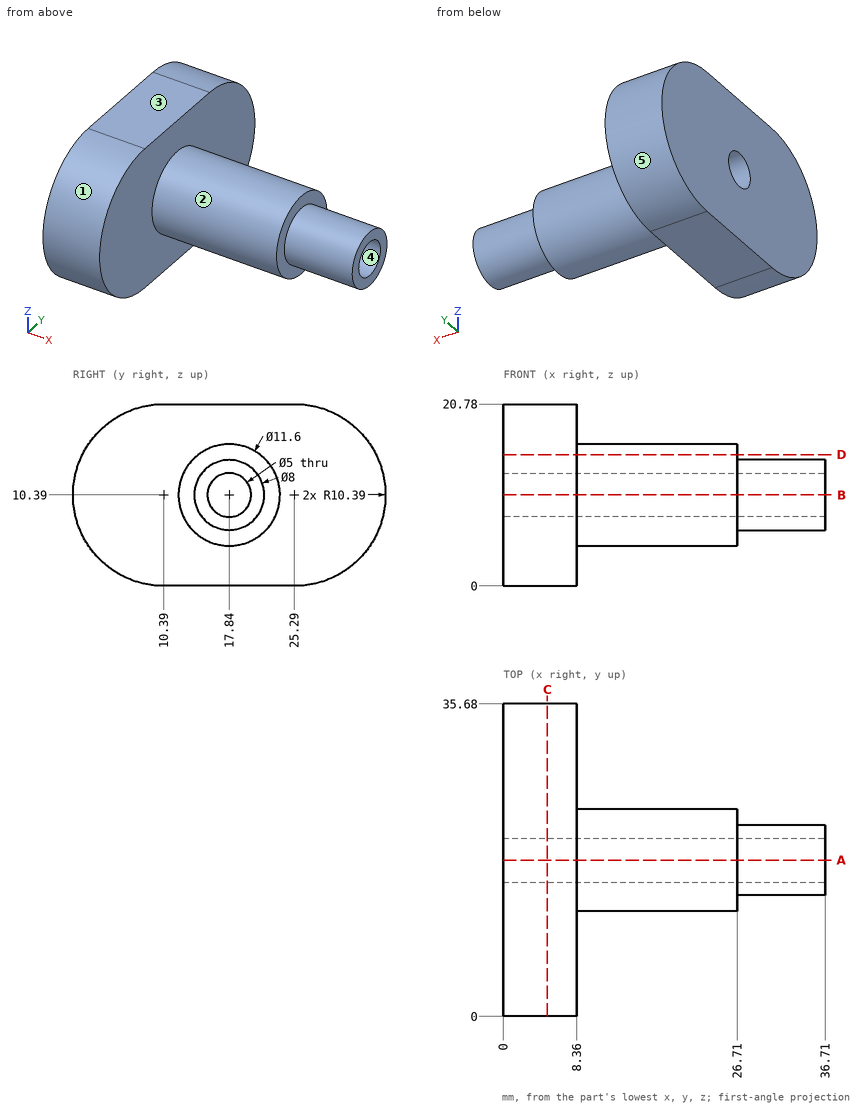
Check sheet for the drawn part. Datum: minimum x, y, z corner. Units: mm. A direction names the side the tool comes from. Coordinates: 2 decimals unless noted, no trailing zeros. Order: outer loops, then holes, each group sorted by start corner. A loop starts at its lowest first (then second) coordinate and runs counter-clockwise, first axis right, second up. Notation, with made-up numbers: (-11.5, 71) -> (39.5, 71) arc R30 cw to (39.5, 98) -> close; hole circle Ø2 at (82.5, 3). An arc over 180 degrees is marked (long way). Use a Markdown table: item, result. Add a question column.
1. Cross-section at C-C (x = 5). Enter the section's corners in (y, z).
2. Set-up check for the marked faces 1 and 2: record each of +Z, -Z, +X, -X, +Y, -Y from which the full face is reachable in a straight line by a thin tool's end or side.
3. Cross-section at A-A (y = 17.84). Enter the section's corners in (x, z).
4. Cross-section at D-D (z = 15). Enter the section's corners in (x, y).
5. Cross-section at B-B (z = 10.39). Enter the section's corners in (x, y), and give its area (3 significant figures).
6. Mould release check, pull along Z, two halves, no side actions. Record for the marked faces 3, 4 and 5: pulls with the +Z half, pulls with the -Z half, needs draft (parallel to the pull), parting line crosses it, or undercut.
7. Go/stop test with flat-tipped pins: pin 1 Ø1.5 at (y, z) = (25.5, 9) entering from +X; pin 2 Ø2 at (x, y) = (27, 14) entering from -Z; pin 3 Ø2 at (x, y) = (31, 11) entering from +Z; pin 4 Ø12 at (x, z) = (4.5, 18) entering from -Y. Record where each tip stops, or that it passes through.
8. Material ranges on L1, parallel to Y at x = 8, z = 10.39; L2, parallel to Y at x = 23, z = 10.39; L3, parallel to X at y = 12.5, z = 4.5, recorded low to high.
Filled sheet:
| question | item | result |
|---|---|---|
| 1 | outline | (10.39, 0) -> (25.29, 0) arc R10.39 ccw to (25.29, 20.78) -> (10.39, 20.78) arc R10.39 ccw to start; hole circle Ø5 at (17.84, 10.39) |
| 2 | face 1 | +X, -X, -Y |
| 2 | face 2 | +X |
| 3 | outline | (0, 0) -> (8.36, 0) -> (8.36, 4.59) -> (26.71, 4.59) -> (26.71, 6.39) -> (36.71, 6.39) -> (36.71, 7.89) -> (0, 7.89) -> close; (0, 12.89) -> (36.71, 12.89) -> (36.71, 14.39) -> (26.71, 14.39) -> (26.71, 16.19) -> (8.36, 16.19) -> (8.36, 20.78) -> (0, 20.78) -> close |
| 4 | outline | (0, 1.08) -> (8.36, 1.08) -> (8.36, 14.32) -> (26.71, 14.32) -> (26.71, 21.36) -> (8.36, 21.36) -> (8.36, 34.6) -> (0, 34.6) -> close |
| 5 | outline | (0, 0) -> (8.36, 0) -> (8.36, 12.04) -> (26.71, 12.04) -> (26.71, 13.84) -> (36.71, 13.84) -> (36.71, 15.34) -> (0, 15.34) -> close; (0, 20.34) -> (36.71, 20.34) -> (36.71, 21.84) -> (26.71, 21.84) -> (26.71, 23.64) -> (8.36, 23.64) -> (8.36, 35.68) -> (0, 35.68) -> close |
| 5 | area | 408 mm2 |
| 6 | face 3 | pulls with the +Z half |
| 6 | face 4 | undercut |
| 6 | face 5 | parting line crosses it |
| 7 | pin 1 | x = 8.36 |
| 7 | pin 2 | z = 5.36 |
| 7 | pin 3 | through |
| 7 | pin 4 | y = 0.13 |
| 8 | L1 | 0 to 15.34, 20.34 to 35.68 |
| 8 | L2 | 12.04 to 15.34, 20.34 to 23.64 |
| 8 | L3 | 0 to 8.36 |
